```python
from build123d import *

# Parameters (mm, degrees)
SKETCH1_W           = 120
SKETCH1_H           = 55
SKETCH1_R           = 3
BOSS_EXTRUDE1_DEPTH = 3
SKETCH2_W           = 20
SKETCH2_H           = 3
BOSS_EXTRUDE2_DEPTH = 3


with BuildPart() as part:
    # Sketch1 → Boss-Extrude1 (new body)
    with BuildSketch(Plane.XY):
        with Locations((60, 27.5)):
            Rectangle(SKETCH1_W, SKETCH1_H)
        with Locations((60, 6)):
            Circle(SKETCH1_R, mode=Mode.SUBTRACT)
    extrude(amount=-BOSS_EXTRUDE1_DEPTH)

    # Sketch2 → Boss-Extrude2 (add)
    with BuildSketch(Plane.XY):
        with Locations((30, -1.5)):
            Rectangle(SKETCH2_W, SKETCH2_H)
        with Locations((90, -1.5)):
            Rectangle(SKETCH2_W, SKETCH2_H)
    extrude(amount=-BOSS_EXTRUDE2_DEPTH)


solid = part.part
```
Can you work these out from the model? Positions are in its coordinate system, mm. A direction names the side the tool comes from. Round coordinates to 2 decimals unless told otherwise and drop trailing zeros. Loops run counter-clockwise (first coordinate to the right, second up) from the corner with the lowest first, then second, coordinate; pieces in that order, holes last. Notation, with made-up numbers: (54, 79.5) -> (83, 79.5) arc R32 cw to (83, 106.5) -> close; hole circle Ø1 at (71, -6.5). An arc over 180 degrees is marked (long way). Answer in a Markdown table with one row per item.
Item 1: Will these pins go through, and if not, where does the flat tip stop? P1, Ø1.5, axis at x = 111.5, z = -1, coming from the -Y side; P2, Ø1.5, axis at y = -1, z = -1.5, coming from the +X side.
Answer block:
| item | result |
|---|---|
| P1 | y = 0 |
| P2 | x = 100 |
Item 2: On a 3-axis mill with a long thin cutter (end or side, diameter ignored), from which of +Z, -Z, +X, -X, +Y, -Y can I reach the whole of each face in a straight line? I mean faces 5 (the flat face through (80, -2, -1)), 6 (the flat face through (110, 0, -1)), 7 (the flat face through (10, 0, -1)), 8 (the cylindrical face through (57, 6, -1)). Say none if no direction works.
Answer block:
| item | result |
|---|---|
| face 5 | +Z, -Z, -Y |
| face 6 | +Z, -Z, +X, -Y |
| face 7 | +Z, -Z, -X, -Y |
| face 8 | +Z, -Z |
Item 3: If I drill on probe 1 along Y at (x, z) = (60, -2.35); probe 2 along Y at (x, z) = (53, -0.7); probe 3 along Y at (x, z) = (62.5, -1.9), over which ranges is the centre line in solid material (lowest first)?
Answer block:
| item | result |
|---|---|
| probe 1 | 0 to 3, 9 to 55 |
| probe 2 | 0 to 55 |
| probe 3 | 0 to 4.34, 7.66 to 55 |
Item 4: Suppose I cut it at A-A, the plane y = 6. List the corners of the cut face in (x, z) for me.
Answer block:
| item | result |
|---|---|
| outline | (0, -3) -> (57, -3) -> (57, 0) -> (0, 0) -> close; (63, -3) -> (120, -3) -> (120, 0) -> (63, 0) -> close |
Item 5: Suppose I cut it at B-B, the plane z = -1.15. List the corners of the cut face in (x, y) for me.
Answer block:
| item | result |
|---|---|
| outline | (0, 0) -> (20, 0) -> (20, -3) -> (40, -3) -> (40, 0) -> (80, 0) -> (80, -3) -> (100, -3) -> (100, 0) -> (120, 0) -> (120, 55) -> (0, 55) -> close; hole circle Ø6 at (60, 6) |
Item 6: Suppose I cut it at D-D, the plane x = 46.5. List the corners of the cut face in (y, z) for me, plus the area to 3 significant figures.
Answer block:
| item | result |
|---|---|
| outline | (0, -3) -> (55, -3) -> (55, 0) -> (0, 0) -> close |
| area | 165 mm² |
Item 7: Suppose I cut it at C-C, the plane x = 60. List the corners of the cut face in (y, z) for me, plus the area to 3 significant figures.
Answer block:
| item | result |
|---|---|
| outline | (0, -3) -> (3, -3) -> (3, 0) -> (0, 0) -> close; (9, -3) -> (55, -3) -> (55, 0) -> (9, 0) -> close |
| area | 147 mm² |
Item 8: We'd pull the mould along X, two halves only. Please class faces 1 (the flat face through (20, -2, -1)), 2 (the flat face through (40, -2, -1)), 3 (the flat face through (60, 0, -1)), 4 (the flat face through (120, 27, -1)): released by +X, released by -X, zero draft, split by the parting line, or undercut.
Answer block:
| item | result |
|---|---|
| face 1 | released by -X |
| face 2 | undercut |
| face 3 | undercut |
| face 4 | released by +X |
